from build123d import *

# Parameters (mm, degrees)
F3_DEPTH = 2250
F4_DEPTH = 63.5
F5_W     = 62
F5_H     = 3.5
F5_H_2   = 27.5
F6_DEPTH = 25
F8_DEPTH = 80
F9_R     = 3.5


with BuildPart() as f3:
    # F2 (on Front) → F3 (new body)
    with BuildSketch(Plane.XZ):
        with BuildLine():
            ThreePointArc((32.5, 27.5), (31.0355339059, 31.0355339059), (27.5, 32.5))
            Line((27.5, 32.5), (-27.5, 32.5))
            ThreePointArc((-27.5, 32.5), (-31.0355339059, 31.0355339059), (-32.5, 27.5))
            Line((-32.5, 27.5), (-32.5, -27.5))
            ThreePointArc((-32.5, -27.5), (-31.0355339059, -31.0355339059), (-27.5, -32.5))
            Line((-27.5, -32.5), (27.5, -32.5))
            ThreePointArc((27.5, -32.5), (31.0355339059, -31.0355339059), (32.5, -27.5))
            Line((32.5, -27.5), (32.5, 27.5))
        make_face()
        with BuildLine():
            ThreePointArc((27.5, 31), (29.9748737342, 29.9748737342), (31, 27.5))
            Line((31, 27.5), (31, -27.5))
            ThreePointArc((31, -27.5), (29.9748737342, -29.9748737342), (27.5, -31))
            Line((27.5, -31), (-27.5, -31))
            ThreePointArc((-27.5, -31), (-29.9748737342, -29.9748737342), (-31, -27.5))
            Line((-31, -27.5), (-31, 27.5))
            ThreePointArc((-31, 27.5), (-29.9748737342, 29.9748737342), (-27.5, 31))
            Line((-27.5, 31), (27.5, 31))
        make_face(mode=Mode.SUBTRACT)
    extrude(amount=F3_DEPTH)

    # F2 (on Front) → F4 (join, symmetric)
    with BuildSketch(Plane.XZ):
        with BuildLine():
            Line((31, -27.5), (31, 27.5))
            ThreePointArc((31, 27.5), (29.9748737342, 29.9748737342), (27.5, 31))
            Line((27.5, 31), (-27.5, 31))
            ThreePointArc((-27.5, 31), (-29.9748737342, 29.9748737342), (-31, 27.5))
            Line((-31, 27.5), (-31, -27.5))
            ThreePointArc((-31, -27.5), (-29.9748737342, -29.9748737342), (-27.5, -31))
            Line((-27.5, -31), (27.5, -31))
            ThreePointArc((27.5, -31), (29.9748737342, -29.9748737342), (31, -27.5))
        make_face()
    extrude(amount=F4_DEPTH, both=True)

    # F5 (on face) → F6 (join)
    with BuildSketch(Plane.YZ.offset(31)):
        with Locations((32.5, 29.25)):
            Rectangle(F5_W, F5_H)
        with Locations((32.5, 13.75)):
            Rectangle(F5_W, F5_H_2)
        with Locations((32.5, -13.75)):
            Rectangle(F5_W, F5_H_2)
        with Locations((32.5, -29.25)):
            Rectangle(F5_W, F5_H)
    extrude(amount=-F6_DEPTH)

    # F7 (on face) → F8 (join)
    with BuildSketch(Plane.YZ.offset(31)):
        Polygon((63.5, 31), (1.5, 31), (1.5, 27.5), (1.5, -27.5), (1.5, -31), (63.5, -31), align=None)
    extrude(amount=F8_DEPTH)

    # F9
    f9_edges = [f3.edges().sort_by_distance(p)[0] for p in [
        (41.75, 63.5, 31),
        (69.25, 1.5, 31),
        (69.25, 1.5, -31),
        (111, 1.5, 0),
        (111, 32.5, -31),
        (111, 63.5, 0),
        (111, 32.5, 31),
        (41.75, 63.5, -31),
    ]]
    fillet(f9_edges, radius=F9_R)


solid = f3.part
Can you work these out from the model? Positions are in its coordinate system, mm. A direction names the side the tool comes from. Give positions to 0.01 mm unless a question says otherwise; leave off trailing zeros. Order: outer loops, then holes, each group sorted by start corner. A loop starts at its lowest first (then second) coordinate and runs counter-clockwise, first axis right, second up. Notation, with made-up numbers: M 35.25,-17.5 L 56.25,-17.5 A31 cw 56.25,21.5 Z; hole C 46.25,55 d5. An arc over 180 degrees is marked long. Use a Markdown table: item, result. Add a question column.
Item 1: Suppose I cut it at B-B (y = -902). List the corners of the cut face in (x, z) for me, then the cut area to 3 significant figures.
Item 2: For faces 4 (the flat face through (32.5, -1109, 0)), 5 (the flat face through (0, -1141, -31)), 6 (the flat face through (39, 30, 31)), which set-ups out of +Z, -Z, +X, -X, +Y, -Y let a thin tool reach every point of the face, with its end or its side?
Item 3: Suppose I cut it at C-C (z = -10.5). List the corners of the cut face in (x, y) for me.
Item 4: We'd pull the mould along X, two halves only. Please class faces 1 (the flat face through (0, -1109, 32.5)), 2 (the flat face through (-32.5, -1109, 0)), 3 (the flat face through (0, -63.5, 0)): +X half, -X half, draft (parallel to the pull), parting line (faces both ways), or undercut.
Item 5: If I drill on L1, parallel to X at y = -815, z = 29; L2, parallel to X at y = -757, z = -13.5, over which ranges is the centre line in solid material (lowest first)? Write a range as [from, to].
Item 6: Will these pins go through, and if not, where does the flat tip stop? pin 1 (16.5 mm diameter, centred on y = -808.5, z = -2.5, fed in from +X); pin 2 (18 mm diameter, centred on x = 69, y = 23.5, fed in from -Z); pin 3 (16.5 mm diameter, centred on y = 20.5, z = 7.5, fed in from -X).
Item 7: Suppose I cut it at A-A (x = -2.5). List the corners of the cut face in (y, z) for me.
Answer sheet:
| question | item | result |
|---|---|---|
| 1 | outline | M -32.5,-27.5 A5 ccw -27.5,-32.5 L 27.5,-32.5 A5 ccw 32.5,-27.5 L 32.5,27.5 A5 ccw 27.5,32.5 L -27.5,32.5 A5 ccw -32.5,27.5 Z; hole M -31,-27.5 A3.5 ccw -27.5,-31 L 27.5,-31 A3.5 ccw 31,-27.5 L 31,27.5 A3.5 ccw 27.5,31 L -27.5,31 A3.5 ccw -31,27.5 Z |
| 1 | area | 370 mm² |
| 2 | face 4 | +Z, -Z, +X, -Y |
| 2 | face 5 | -Y |
| 2 | face 6 | +Z, +X, -X, +Y |
| 3 | outline | M -32.5,-2250 L -31,-2250 L -31,-63.5 L 31,-63.5 L 31,-2250 L 32.5,-2250 L 32.5,0 L 31,0 L 31,1.5 L 107.5,1.5 A3.5 ccw 111,5 L 111,60 A3.5 ccw 107.5,63.5 L -27.5,63.5 A3.5 ccw -31,60 L -31,0 L -32.5,0 Z |
| 4 | face 1 | draft |
| 4 | face 2 | -X half |
| 4 | face 3 | undercut |
| 5 | L1 | x = [-32.27, -30.66], [30.66, 32.27] |
| 5 | L2 | x = [-32.5, -31], [31, 32.5] |
| 6 | pin 1 | stops at x = 32.5 |
| 6 | pin 2 | stops at z = -31 |
| 6 | pin 3 | stops at x = -31 |
| 7 | outline | M -2250,-32.5 L 0,-32.5 L 0,-31 L 60,-31 A3.5 ccw 63.5,-27.5 L 63.5,27.5 A3.5 ccw 60,31 L 0,31 L 0,32.5 L -2250,32.5 L -2250,31 L -63.5,31 L -63.5,-31 L -2250,-31 Z |
